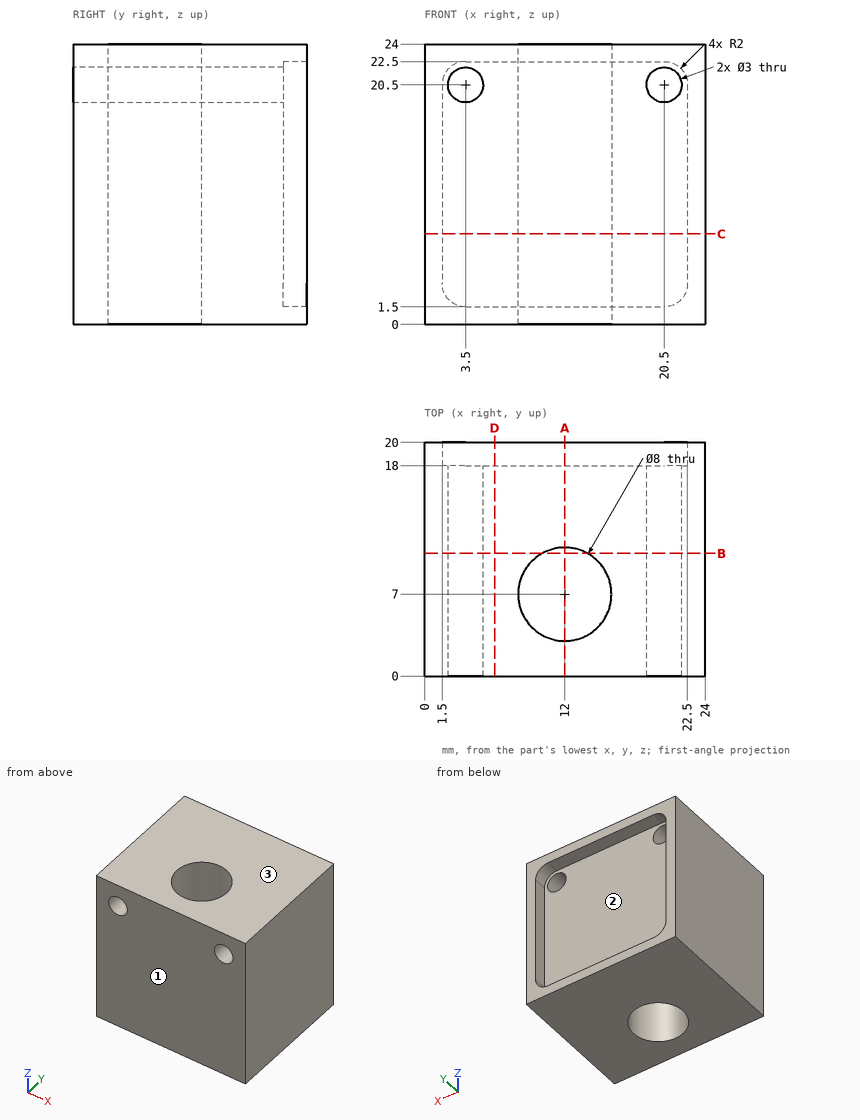
Geometry check sheet. Reference: drawing and pictorial views, mm from the part's lowest x, y, z. Coordinates: 2 decimals unless noted, no trailing zeros. Order: outer loops, then holes, each group sorted by start corner. A loop starts at its lowest first (then second) coordinate and runs counter-clockwise, first axis right, second up. Notation, with made-up numbers: (-37.5, 8.25) -> (21.5, 8.25) arc R12 ccw to (21.5, 26.25) -> close; hole circle Ø9 at (-14, 64.25). An arc over 180 degrees is marked (long way). Put each result on its own line as item: value. Start each with the question number.
1) Cross-section at D-D (x = 6). Enter the section's corners in (y, z).
2) Cross-section at C-C (z = 7.75). Enter the section's corners in (x, y), plus the area to 3 significant figures.
3) Cross-section at A-A (x = 12). Enter the section's corners in (y, z), plus the area to 3 significant figures.
4) Release check for a two-part mould opening along Z. For the marked faces 1, 2 and 3 record: pulls with the +Z half, pulls with the -Z half, needs draft (parallel to the pull), parting line crosses it, or undercut.
5) Cross-section at B-B (y = 10.5). Enter the section's corners in (x, z).
6) Material ranges on L1, parallel to Y at x = 12.25, z = 21.5; L2, parallel to X at y = 4, z = 20.5; L3, parallel to Y at x = 4, z = 12, recorded low to high.
7) Go/stop test with a flat-tipped pin: pin 1 (6.5 mm diameter, centred on x = 8.5, z = 16.5, fed in from +Y). Record where the tip stops, or that it passes through.
Geometry check:
1. outline: (0, 0) -> (20, 0) -> (20, 1.5) -> (18, 1.5) -> (18, 22.5) -> (20, 22.5) -> (20, 24) -> (0, 24) -> close
2. outline: (0, 0) -> (24, 0) -> (24, 20) -> (22.5, 20) -> (22.5, 18) -> (1.5, 18) -> (1.5, 20) -> (0, 20) -> close; hole circle Ø8 at (12, 7)
2. area: 388 mm^2
3. outline: (0, 0) -> (3, 0) -> (3, 24) -> (0, 24) -> close; (11, 0) -> (20, 0) -> (20, 1.5) -> (18, 1.5) -> (18, 22.5) -> (20, 22.5) -> (20, 24) -> (11, 24) -> close
3. area: 246 mm^2
4. face 1: needs draft
4. face 2: undercut
4. face 3: pulls with the +Z half
5. outline: (0, 0) -> (10.06, 0) -> (10.06, 24) -> (0, 24) -> close; (13.94, 0) -> (24, 0) -> (24, 24) -> (13.94, 24) -> close; hole circle Ø3 at (3.5, 20.5); hole circle Ø3 at (20.5, 20.5)
6. L1: y = 0 to 3.01, 10.99 to 18
6. L2: x = 0 to 2, 5 to 9.35, 14.65 to 19, 22 to 24
6. L3: y = 0 to 18
7. pin 1: stops at y = 18
